Build history of the part. All positions in model axes, mm. Round coordinates to 2 decimals unless told otherwise and drop trailing zeros. Write each loop counter-clockwise with the first axis right and the second up, starting at its lowest first coordinate (ties: lowest second). Pieces come first, ordered by that corner, then holes. Notation, with made-up numbers: (-16, 31) -> (24, 31) arc R24 ccw to (24, 60) -> close; hole circle Ø5 at (-35, 67). An arc over 180 degrees is marked (long way). One line per question, with ' | ' between items.
from build123d import *

# Parameters (mm, degrees)
SKETCH1_W             = 80
SKETCH1_H             = 225
BOSS_EXTRUDE1_DEPTH   = 10
CUT_EXTRUDE1_REACH    = 121.818
SKETCH2_R             = 6
M8_CLEARANCE_HOLE1_D  = 8.4
F_8_0MM_DOWEL_HOLE1_D = 8
CUT_EXTRUDE3_REACH    = 121.818
SKETCH10_R            = 7
SKETCH14_R            = 10
CUT_EXTRUDE4_DEPTH    = 120.817569663


with BuildPart() as part:
    # Sketch1 → Boss-Extrude1 (new body)
    with BuildSketch(Plane(origin=(0, 0, 0), x_dir=(1, 0, 0), z_dir=(0, 1, 0))):
        Rectangle(SKETCH1_W, SKETCH1_H)
    extrude(amount=-BOSS_EXTRUDE1_DEPTH)

    # Sketch2 → Cut-Extrude1 (cut, up to next)
    with BuildSketch(Plane(origin=(0, 0, 0), x_dir=(1, 0, 0), z_dir=(0, 1, 0)), mode=Mode.PRIVATE) as cut_extrude1_sk1:
        with Locations(Location((0, 100, 0), (0, 0, 270))):
            Circle(SKETCH2_R)
    cut_extrude1_tool1 = extrude(cut_extrude1_sk1.sketch, amount=-CUT_EXTRUDE1_REACH, mode=Mode.PRIVATE) & part.part
    # Sketch2 → Cut-Extrude1 (cut, up to next)
    with BuildSketch(Plane(origin=(0, 0, 0), x_dir=(1, 0, 0), z_dir=(0, 1, 0)), mode=Mode.PRIVATE) as cut_extrude1_sk2:
        with Locations(Location((30, 4, 0), (0, 0, 270))):
            Circle(SKETCH2_R)
    cut_extrude1_tool2 = extrude(cut_extrude1_sk2.sketch, amount=-CUT_EXTRUDE1_REACH, mode=Mode.PRIVATE) & part.part
    # Sketch2 → Cut-Extrude1 (cut, up to next)
    with BuildSketch(Plane(origin=(0, 0, 0), x_dir=(1, 0, 0), z_dir=(0, 1, 0)), mode=Mode.PRIVATE) as cut_extrude1_sk3:
        with Locations(Location((-30, 4, 0), (0, 0, 270))):
            Circle(SKETCH2_R)
    cut_extrude1_tool3 = extrude(cut_extrude1_sk3.sketch, amount=-CUT_EXTRUDE1_REACH, mode=Mode.PRIVATE) & part.part
    # Sketch2 → Cut-Extrude1 (cut, up to next)
    with BuildSketch(Plane(origin=(0, 0, 0), x_dir=(1, 0, 0), z_dir=(0, 1, 0)), mode=Mode.PRIVATE) as cut_extrude1_sk4:
        with Locations(Location((0, -100, 0), (0, 0, 270))):
            Circle(SKETCH2_R)
    cut_extrude1_tool4 = extrude(cut_extrude1_sk4.sketch, amount=-CUT_EXTRUDE1_REACH, mode=Mode.PRIVATE) & part.part
    add(cut_extrude1_tool1.solids().sort_by_distance((0, 0, -100))[0], mode=Mode.SUBTRACT)
    add(cut_extrude1_tool2.solids().sort_by_distance((30, 0, -4))[0], mode=Mode.SUBTRACT)
    add(cut_extrude1_tool3.solids().sort_by_distance((-30, 0, -4))[0], mode=Mode.SUBTRACT)
    add(cut_extrude1_tool4.solids().sort_by_distance((0, 0, 100))[0], mode=Mode.SUBTRACT)

    # M8 Clearance Hole1 (through all)
    with Locations(Plane(origin=(0, 0, 0), x_dir=(1, 0, 0), z_dir=(0, 1, 0))):
        with Locations((-25, 97.5), (25, 97.5), (25, -97.5), (-25, -97.5)):
            Hole(M8_CLEARANCE_HOLE1_D / 2)

    # Ø8.0mm Dowel Hole1 (through all)
    with Locations(Plane(origin=(0, 0, 0), x_dir=(1, 0, 0), z_dir=(0, 1, 0))):
        with Locations((25, 81.975), (-25, -82)):
            Hole(F_8_0MM_DOWEL_HOLE1_D / 2)

    # Sketch10 → Cut-Extrude3 (cut, up to next)
    with BuildSketch(Plane(origin=(0, 0, 0), x_dir=(1, 0, 0), z_dir=(0, 1, 0)), mode=Mode.PRIVATE) as cut_extrude3_sk1:
        with Locations(Location((0, 9.86, 0), (0, 0, 270))):
            Circle(SKETCH10_R)
    cut_extrude3_tool1 = extrude(cut_extrude3_sk1.sketch, amount=-CUT_EXTRUDE3_REACH, mode=Mode.PRIVATE) & part.part
    add(cut_extrude3_tool1.solids().sort_by_distance((0, 0, -9.86))[0], mode=Mode.SUBTRACT)

    # Sketch14 → Cut-Extrude4 (cut, through all)
    with BuildSketch(Plane(origin=(0, -10, 0), x_dir=(1, 0, 0), z_dir=(0, 1, 0))):
        with Locations(Location((22, 60, 0), (0, 0, 270))):
            Circle(SKETCH14_R)
        with Locations(Location((-22, 72, 0), (0, 0, 270))):
            Circle(SKETCH14_R)
        with Locations(Location((0, 35, 0), (0, 0, 270))):
            Circle(SKETCH14_R)
        with Locations(Location((0, -25, 0), (0, 0, 270))):
            Circle(SKETCH14_R)
        with Locations(Location((-22, -55, 0), (0, 0, 270))):
            Circle(SKETCH14_R)
        with Locations(Location((22, -55, 0), (0, 0, 270))):
            Circle(SKETCH14_R)
    extrude(amount=CUT_EXTRUDE4_DEPTH, mode=Mode.SUBTRACT)


solid = part.part
(1) Wall check: line 1 (X direction, y = -2.5, z = 25); line 2 (Z direction, x = 1, y = -4.5); line 3 (X direction, y = -3.25, z = -97.5). Give the ranges that are in metal, low to high. Write a range as from..to.
Calculated:
line 1: -40..-10, 10..40 | line 2: -112.5..-105.92, -94.08..-44.95, -25.05..-16.79, -2.93..15.05, 34.95..94.08, 105.92..112.5 | line 3: -40..-29.2, -20.8..-5.45, 5.45..20.8, 29.2..40
(2) Slice it at A-A (z = -60). Write the cut outline in (x, y).
Calculated:
outline: (-40, -10) -> (12, -10) -> (12, 0) -> (-40, 0) -> close; (32, -10) -> (40, -10) -> (40, 0) -> (32, 0) -> close
(3) Slice it at D-D (z = 82). Write the cut outline in (x, y), then the cut area to 3 significant figures.
Calculated:
outline: (-40, -10) -> (-29, -10) -> (-29, 0) -> (-40, 0) -> close; (-21, -10) -> (40, -10) -> (40, 0) -> (-21, 0) -> close | area: 720 mm2
(4) Mould opens along X. For faces 1 (the flat face through (-40, -5, 2)), 2 (the flat face through (40, -5, 2)), 3 (the cylindrical face through (0, -5, -45)), 4 (the cylindrical face through (-24.133, -5.07, 85.905)) say: pulls with the +X half, pulls with the -X half, needs draft (parallel to the pull), parting line crosses it, or undercut.
Calculated:
face 1: pulls with the -X half | face 2: pulls with the +X half | face 3: undercut | face 4: undercut
(5) Slice it at C-C (z = -97.5). Write the cut outline in (x, y), then the cut area to 3 significant figures.
Calculated:
outline: (-40, -10) -> (-29.2, -10) -> (-29.2, 0) -> (-40, 0) -> close; (-20.8, -10) -> (-5.45, -10) -> (-5.45, 0) -> (-20.8, 0) -> close; (5.45, -10) -> (20.8, -10) -> (20.8, 0) -> (5.45, 0) -> close; (29.2, -10) -> (40, -10) -> (40, 0) -> (29.2, 0) -> close | area: 523 mm2
(6) Slice it at B-B (y = -1.5). State how many separate pieces and enclosed holes the cut face has, then the cut area to 3 significant figures.
Calculated:
separate pieces: 1 | enclosed holes: 17 | area: 15,200 mm2
